```python
from build123d import *

# Parameters (mm, degrees)
RESSALTO_EXTRUS_O1_DEPTH = 6
FILETE1_R                = 1


with BuildPart() as part:
    # Esboço2 → Ressalto-extrusão1 (new body)
    with BuildSketch(Plane(origin=(0, 0, 0), x_dir=(1, 0, 0), z_dir=(0, 1, 0))):
        with BuildLine():
            Line((-11.375, -102.828494661), (-11.375, -41.212577741))
            ThreePointArc((-11.375, -41.212577741), (-8.710783638, -27.818657608), (-1.123737342, -16.463840399))
            Line((-1.123737342, -16.463840399), (27.30266953, 11.962566472))
            ThreePointArc((27.30266953, 11.962566472), (32.721988313, 20.073150192), (34.625, 29.640236002))
            Line((34.625, 29.640236002), (34.625, 121.17150534))
            Line((34.625, 121.17150534), (39.625, 121.17150534))
            Line((39.625, 121.17150534), (39.625, 29.640236002))
            ThreePointArc((39.625, 29.640236002), (37.341385975, 18.159733031), (30.838203436, 8.427032566))
            Line((30.838203436, 8.427032566), (2.411796564, -19.999374305))
            ThreePointArc((2.411796564, -19.999374305), (-4.091385975, -29.73207477), (-6.375, -41.212577741))
            Line((-6.375, -41.212577741), (-6.375, -102.828494661))
            Line((-6.375, -102.828494661), (-11.375, -102.828494661))
        make_face()
    extrude(amount=RESSALTO_EXTRUS_O1_DEPTH)

    # Filete1
    filete1_edges = [part.edges().sort_by_distance(p)[0] for p in [
        (39.625, 0, -75.405870671),
        (37.341385975, 0, -18.159733031),
        (32.721988313, 6, -20.073150192),
        (16.625, 0, 5.78617087),
        (-4.091385975, 0, 29.73207477),
        (-6.375, 0, 72.020536201),
        (-11.375, 0, 72.020536201),
        (-8.710783638, 0, 27.818657608),
        (13.089466094, 0, 2.250636964),
        (32.721988313, 0, -20.073150192),
        (34.625, 0, -75.405870671),
        (13.089466094, 6, 2.250636964),
        (-8.710783638, 6, 27.818657608),
        (-11.375, 3, 102.828494661),
        (34.625, 3, -121.17150534),
        (-11.375, 6, 72.020536201),
        (-6.375, 6, 72.020536201),
        (-4.091385975, 6, 29.73207477),
        (16.625, 6, 5.78617087),
        (37.341385975, 6, -18.159733031),
        (39.625, 6, -75.405870671),
        (34.625, 6, -75.405870671),
    ]]
    fillet(filete1_edges, radius=FILETE1_R)


solid = part.part
```
Geometry check sheet. Reference: the model listing, model coordinates, mm. A direction names the side the tool comes from. Coordinates: 2 decimals unless noted, no trailing zeros. Write each loop counter-clockwise with the first axis right and the second up, starting at its lowest first coordinate (ties: lowest second). Pieces come first, ordered by that corner, then holes. Notation, with made-up numbers: M 75,-25.75 L 116,-25.75 A11 ccw 116,-20.75 Z; hole C 25,22.5 d8. An arc over 180 degrees is marked long. Use one line per item in the form item = value. Start each with the question number.
1) Section check A-A on y = 2.65. Enter the section's corners in (x, z) (1 decimal), and give its area (3 significant figures).
2) Thickness scan on probe 1 along X at (y, z) = (4.2, -102) (3 decimals); probe 2 along X at (y, z) = (4.4, 54) (3 decimals); probe 3 along Z at (x, y) = (-3, 0.5). Record the ranges inside material, lowest first. Write a range as from..to.
3) Section check B-B on z = -65. Enter the section's corners in (x, y) (3 decimals).
4) Set-up check for faces 1 (the flat face through (34.625, 3, -74)), 2 (the flat face through (-6.375, 3, 72)), 3 (the flat face through (38, 3, -121.172)): record each of +Z, -Z, +X, -X, +Y, -Y from which the full face is reachable in a straight line by a thin tool's end or side.
5) Go/stop test with flat-tipped pins: pin 1 Ø3 at (y, z) = (3, 29) entering from +X; pin 2 Ø1 at (y, z) = (1, 61.5) entering from +X (3 decimals); pin 3 Ø1 at (x, y) = (9.5, 2) entering from +Z. Record where each tip stops, or that it passes through.
Responses:
q1.outline = M -11.4,41.2 A35 ccw -1.1,16.5 L 27.3,-12 A25 cw 34.6,-29.6 L 34.6,-120.2 A1 ccw 35.6,-121.2 L 39.6,-121.2 L 39.6,-29.6 A30 ccw 30.8,-8.4 L 2.4,20 A30 cw -6.4,41.2 L -6.4,102.8 L -10.4,102.8 A1 ccw -11.4,101.8 Z
q1.area = 1,200 mm2
q2.probe_1 = 34.625..39.625
q2.probe_2 = -11.375..-6.375
q2.probe_3 = 18.7..27.1
q3.outline = M 34.625,1 A1 ccw 35.625,0 L 38.625,0 A1 ccw 39.625,1 L 39.625,5 A1 ccw 38.625,6 L 35.625,6 A1 ccw 34.625,5 Z
q4.face_1 = -Z, -X, +Y, -Y
q4.face_2 = +Z, +X, +Y, -Y
q4.face_3 = -Z, +X, -X, +Y, -Y
q5.pin_1 = -3.06
q5.pin_2 = -6.375
q5.pin_3 = 13.41
